Could you check a few things on this drawing? It's one solid part, dimensions in mm from its lowest x, y, z. A direction names the side the tool comes from. Coordinates: 2 decimals unless noted, no trailing zeros. Loops run counter-clockwise (first coordinate to the right, second up) from the corner with the lowest first, then second, coordinate; pieces in that order, holes last. Notation, with made-up numbers: (-37.5, 49) -> (-7.5, 49) arc R13 ccw to (-7.5, 66) -> close; hole circle Ø11 at (48.25, 89). An arc over 180 degrees is marked (long way). One line per question, with ' | ' between items.
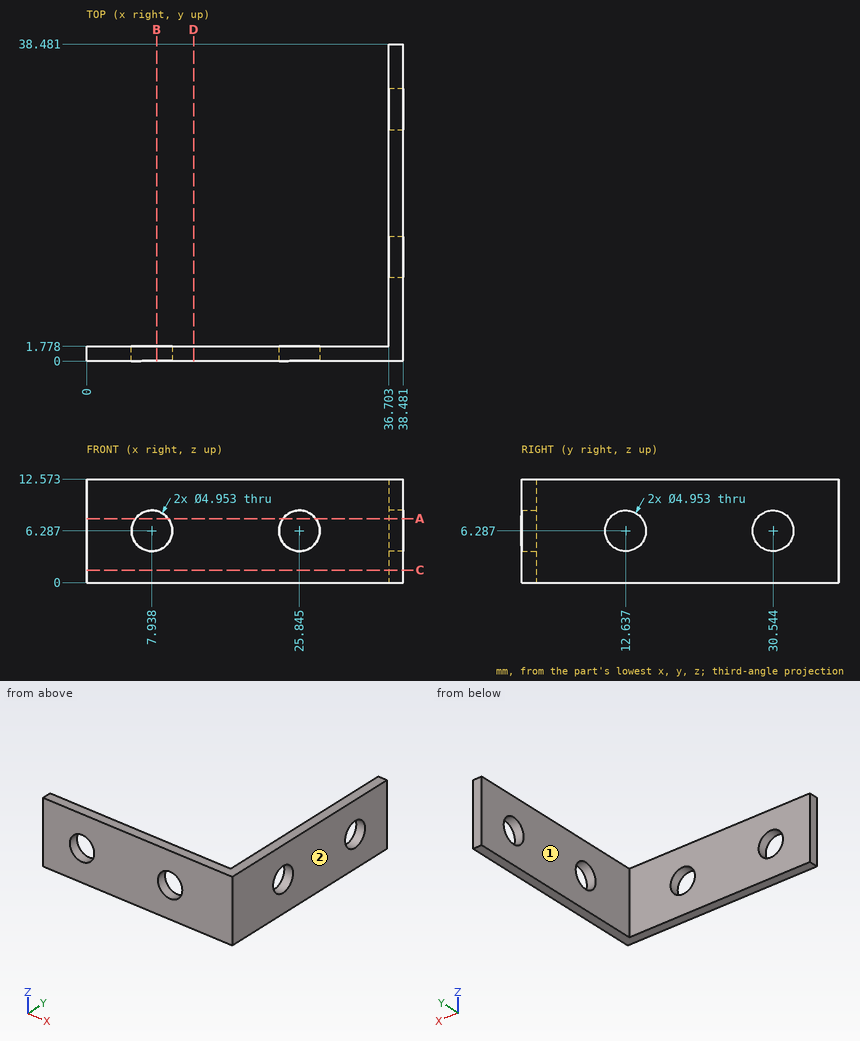
1) If we section it at C-C on z = 1.5: Please give me the cut outline in (x, y), and give its area (3 significant figures).
Data:
outline: (0, 0) -> (38.48, 0) -> (38.48, 38.48) -> (36.7, 38.48) -> (36.7, 1.78) -> (0, 1.78) -> close | area: 134 mm²
2) On a 3-axis mill with a long thin cutter (end or side, diameter ignored), from which of +Z, -Z, +X, -X, +Y, -Y can I reach the whole of each face in a straight line? I mean the marked faces 1 and 2. Say none if no direction works.
Data:
face 1: +Z, -Z, -X, +Y | face 2: +Z, -Z, +X, +Y, -Y
3) I need wall thicknesses on line 1 along X through (y, z) = (4, 10); line 2 along Y through (x, z) = (32, 7.25). Which ranges of each line are inside material? Lowest first, please. Write a range as from..to.
Data:
line 1: 36.7..38.48 | line 2: 0..1.78
4) If we section it at B-B on x = 8.5: Please give me the cut outline in (y, z) (1 decimal), and give its area (3 significant figures).
Data:
outline: (0, 0) -> (1.8, 0) -> (1.8, 3.9) -> (0, 3.9) -> close; (0, 8.7) -> (1.8, 8.7) -> (1.8, 12.6) -> (0, 12.6) -> close | area: 13.8 mm²
5) I'm going to push flat-ended pins straight in: pin 1 Ø1.5 at (y, z) = (21.5, 4.5) entering from -X; pin 2 Ø1.5 at (x, z) = (27.5, 11) entering from +Y. Where does each tip first touch, or does it pass through?
Data:
pin 1: x = 36.7 | pin 2: y = 1.78
6) If we section it at D-D on x = 13: Please give me the cut outline in (y, z).
Data:
outline: (0, 0) -> (1.78, 0) -> (1.78, 12.57) -> (0, 12.57) -> close
7) If we section it at A-A on z = 7.75: Please give me the cut outline in (x, y) (1 decimal), and give its area (3 significant figures).
Data:
outline: (0, 0) -> (5.9, 0) -> (5.9, 1.8) -> (0, 1.8) -> close; (9.9, 0) -> (23.8, 0) -> (23.8, 1.8) -> (9.9, 1.8) -> close; (27.8, 0) -> (38.5, 0) -> (38.5, 10.6) -> (36.7, 10.6) -> (36.7, 1.8) -> (27.8, 1.8) -> close; (36.7, 14.6) -> (38.5, 14.6) -> (38.5, 28.5) -> (36.7, 28.5) -> close; (36.7, 32.5) -> (38.5, 32.5) -> (38.5, 38.5) -> (36.7, 38.5) -> close | area: 105 mm²
